from build123d import *

# Parameters (mm, degrees)
F0_R     = 1.5
F1_DEPTH = 2
F2_R     = 5


with BuildPart() as f1:
    # F0 (on Top) → F1 (new body)
    with BuildSketch(Plane.XY):
        with BuildLine():
            add(Edge.make_bspline(
                [(-13.142859, 26.857141), (-8.951076, 24.20284), (-4.564468, 21.895542), (0, 20)],
                knots=[66.18026, 66.18026, 66.18026, 66.18026, 80.865454, 80.865454, 80.865454, 80.865454], degree=3))
            Line((-13.142859, 26.857141), (-20, 20))
            Line((-20, 20), (-26.857141, 13.142859))
            add(Edge.make_bspline(
                [(-26.857141, 13.142859), (-24.20284, 8.951076), (-21.895542, 4.564468), (-20, 0)],
                knots=[66.18026, 66.18026, 66.18026, 66.18026, 80.865454, 80.865454, 80.865454, 80.865454], degree=3))
            Line((-20, 0), (-14.625, 0))
            Line((-14.625, 0), (-14.625, 6.5))
            Line((-14.625, 6.5), (-12.875, 6.5))
            Line((-12.875, 6.5), (-12.875, 0))
            Line((-12.875, 0), (0, 0))
            Line((0, 0), (0, 20))
        make_face()
        with Locations((-18, 6.25)):
            Circle(F0_R, mode=Mode.SUBTRACT)
        with Locations((-7.5, 7.5)):
            Circle(F0_R, mode=Mode.SUBTRACT)
        with Locations((-6.25, 18)):
            Circle(F0_R, mode=Mode.SUBTRACT)
        with BuildLine():
            Line((-14.625, 0), (-20, 0))
            add(Edge.make_bspline(
                [(-26.854903, -13.145097), (-24.198754, -8.951027), (-21.891877, -4.563394), (-20, 0)],
                knots=[66.166, 66.166, 66.166, 66.166, 80.865454, 80.865454, 80.865454, 80.865454], degree=3))
            Line((-26.854903, -13.145097), (-20, -20))
            Line((-20, -20), (-13.145097, -26.854903))
            add(Edge.make_bspline(
                [(0, -20), (-4.563394, -21.891877), (-8.951027, -24.198754), (-13.145097, -26.854903)],
                knots=[0, 0, 0, 0, 14.699453, 14.699453, 14.699453, 14.699453], degree=3))
            Line((0, -20), (0, 0))
            Line((0, 0), (-12.875, 0))
            Line((-12.875, 0), (-12.875, -6.5))
            Line((-12.875, -6.5), (-14.625, -6.5))
            Line((-14.625, -6.5), (-14.625, 0))
        make_face()
        with Locations((-6.25, -18)):
            Circle(F0_R, mode=Mode.SUBTRACT)
        with Locations((-18, -6.25)):
            Circle(F0_R, mode=Mode.SUBTRACT)
        with Locations((-7.5, -7.5)):
            Circle(F0_R, mode=Mode.SUBTRACT)
        with BuildLine():
            Line((-11.161165, 28.838835), (-13.142859, 26.857141))
            add(Edge.make_bspline(
                [(-13.142859, 26.857141), (-8.951076, 24.20284), (-4.564468, 21.895542), (0, 20)],
                knots=[66.18026, 66.18026, 66.18026, 66.18026, 80.865454, 80.865454, 80.865454, 80.865454], degree=3))
            add(Edge.make_bspline(
                [(13.145097, 26.854903), (8.951027, 24.198754), (4.563394, 21.891877), (0, 20)],
                knots=[66.166, 66.166, 66.166, 66.166, 80.865454, 80.865454, 80.865454, 80.865454], degree=3))
            Line((13.145097, 26.854903), (11.161165, 28.838835))
            add(Edge.make_bspline(
                [(-11.161165, 28.838835), (-7.440777, 25.169417), (0, 17.830583), (7.440777, 25.169417), (11.161165, 28.838835)],
                knots=[0, 0, 0, 0, 13.357773, 26.715546, 26.715546, 26.715546, 26.715546], degree=3))
        make_face()
        with BuildLine():
            add(Edge.make_bspline(
                [(-26.857141, 13.142859), (-24.20284, 8.951076), (-21.895542, 4.564468), (-20, 0)],
                knots=[66.18026, 66.18026, 66.18026, 66.18026, 80.865454, 80.865454, 80.865454, 80.865454], degree=3))
            Line((-26.857141, 13.142859), (-28.838835, 11.161165))
            add(Edge.make_bspline(
                [(-28.838835, -11.161165), (-25.169417, -7.440777), (-17.830583, 0), (-25.169417, 7.440777), (-28.838835, 11.161165)],
                knots=[0, 0, 0, 0, 13.357773, 26.715546, 26.715546, 26.715546, 26.715546], degree=3))
            Line((-28.838835, -11.161165), (-26.854903, -13.145097))
            add(Edge.make_bspline(
                [(-26.854903, -13.145097), (-24.198754, -8.951027), (-21.891877, -4.563394), (-20, 0)],
                knots=[66.166, 66.166, 66.166, 66.166, 80.865454, 80.865454, 80.865454, 80.865454], degree=3))
        make_face()
        with BuildLine():
            Line((28.838835, 11.161165), (26.854903, 13.145097))
            add(Edge.make_bspline(
                [(26.854903, 13.145097), (24.198754, 8.951027), (21.891877, 4.563394), (20, 0)],
                knots=[66.166, 66.166, 66.166, 66.166, 80.865454, 80.865454, 80.865454, 80.865454], degree=3))
            add(Edge.make_bspline(
                [(20, 0), (21.891877, -4.563394), (24.198754, -8.951027), (26.854903, -13.145097)],
                knots=[0, 0, 0, 0, 14.699454, 14.699454, 14.699454, 14.699454], degree=3))
            Line((26.854903, -13.145097), (28.838835, -11.161165))
            add(Edge.make_bspline(
                [(28.838835, 11.161165), (25.169417, 7.440777), (17.830583, 0), (25.169417, -7.440777), (28.838835, -11.161165)],
                knots=[0, 0, 0, 0, 13.357773, 26.715546, 26.715546, 26.715546, 26.715546], degree=3))
        make_face()
        with BuildLine():
            Line((12.875, 0), (0, 0))
            Line((0, 0), (0, -20))
            add(Edge.make_bspline(
                [(0, -20), (4.563394, -21.891877), (8.951027, -24.198754), (13.145097, -26.854903)],
                knots=[0, 0, 0, 0, 14.699453, 14.699453, 14.699453, 14.699453], degree=3))
            Line((13.145097, -26.854903), (20, -20))
            Line((20, -20), (26.854903, -13.145097))
            add(Edge.make_bspline(
                [(20, 0), (21.891877, -4.563394), (24.198754, -8.951027), (26.854903, -13.145097)],
                knots=[0, 0, 0, 0, 14.699454, 14.699454, 14.699454, 14.699454], degree=3))
            Line((20, 0), (14.625, 0))
            Line((14.625, 0), (14.625, -6.5))
            Line((14.625, -6.5), (12.875, -6.5))
            Line((12.875, -6.5), (12.875, 0))
        make_face()
        with Locations((6.25, -18)):
            Circle(F0_R, mode=Mode.SUBTRACT)
        with Locations((7.5, -7.5)):
            Circle(F0_R, mode=Mode.SUBTRACT)
        with Locations((18, -6.25)):
            Circle(F0_R, mode=Mode.SUBTRACT)
        with BuildLine():
            add(Edge.make_bspline(
                [(0, -20), (4.563394, -21.891877), (8.951027, -24.198754), (13.145097, -26.854903)],
                knots=[0, 0, 0, 0, 14.699453, 14.699453, 14.699453, 14.699453], degree=3))
            add(Edge.make_bspline(
                [(0, -20), (-4.563394, -21.891877), (-8.951027, -24.198754), (-13.145097, -26.854903)],
                knots=[0, 0, 0, 0, 14.699453, 14.699453, 14.699453, 14.699453], degree=3))
            Line((-13.145097, -26.854903), (-11.161165, -28.838835))
            add(Edge.make_bspline(
                [(11.161165, -28.838835), (7.440777, -25.169417), (0, -17.830583), (-7.440777, -25.169417), (-11.161165, -28.838835)],
                knots=[0, 0, 0, 0, 13.357773, 26.715546, 26.715546, 26.715546, 26.715546], degree=3))
            Line((11.161165, -28.838835), (13.145097, -26.854903))
        make_face()
        with BuildLine():
            add(Edge.make_bspline(
                [(13.145097, 26.854903), (8.951027, 24.198754), (4.563394, 21.891877), (0, 20)],
                knots=[66.166, 66.166, 66.166, 66.166, 80.865454, 80.865454, 80.865454, 80.865454], degree=3))
            Line((0, 20), (0, 0))
            Line((0, 0), (12.875, 0))
            Line((12.875, 0), (12.875, 6.5))
            Line((12.875, 6.5), (14.625, 6.5))
            Line((14.625, 6.5), (14.625, 0))
            Line((14.625, 0), (20, 0))
            add(Edge.make_bspline(
                [(26.854903, 13.145097), (24.198754, 8.951027), (21.891877, 4.563394), (20, 0)],
                knots=[66.166, 66.166, 66.166, 66.166, 80.865454, 80.865454, 80.865454, 80.865454], degree=3))
            Line((26.854903, 13.145097), (20, 20))
            Line((20, 20), (13.145097, 26.854903))
        make_face()
        with Locations((7.5, 7.5)):
            Circle(F0_R, mode=Mode.SUBTRACT)
        with Locations((18, 6.25)):
            Circle(F0_R, mode=Mode.SUBTRACT)
        with Locations((6.25, 18)):
            Circle(F0_R, mode=Mode.SUBTRACT)
    extrude(amount=F1_DEPTH)

    # F2
    f2_edges = [f1.edges().sort_by_distance(p)[0] for p in [
        (-11.161165, 28.838835, 1),
        (-28.838835, 11.161165, 1),
        (11.161165, 28.838835, 1),
        (28.838835, 11.161165, 1),
        (28.838835, -11.161165, 1),
        (11.161165, -28.838835, 1),
        (-11.161165, -28.838835, 1),
        (-28.838835, -11.161165, 1),
    ]]
    fillet(f2_edges, radius=F2_R)


solid = f1.part
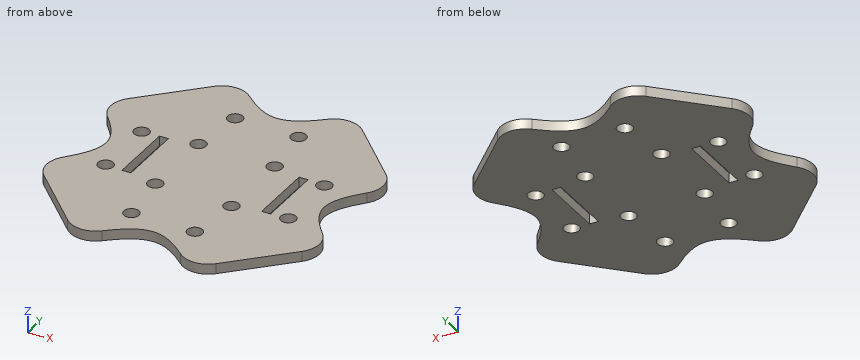
Geometry: final body of the model. Coordinates: model frame, mm. Coordinates: 2 decimals unless noted, no trailing zeros. Order: outer loops, then holes, each group sorted by start corner. A loop starts at its lowest first (then second) coordinate and runs counter-clockwise, first axis right, second up.
(1) Material intervals for probe 1 along X at (y, z) = (-1, 0.55) (3 decimals); probe 2 along X at (y, z) = (-7, 0.45); probe 3 along Y at (x, z) = (17.5, 1.05), sorted ascending.
(2) Section query C-C (z = 0.55). State how many separate pieces and enclosed holes the cut face has, plus the area to 3 significant figures.
(3) Section query A-A (x = -18). Return the cut outline in (y, z), plus the area to 3 significant figures.
(4) First-contact query: pin 1 (0.9 mm diameter, centred on x = 13.5, z = 1, fed in from +Y); pin 2 (0.9 mm diameter, centred on x = 14, z = 1, fed in from -Y). Flat tips, straight axial feed; report the tip coordinate or a pass-through.
Solution:
1. probe 1: x = -21.586 to -14.625, -12.875 to 12.875, 14.625 to 21.586
1. probe 2: x = -24.92 to -19.3, -16.7 to -8.91, -6.09 to 6.09, 8.91 to 16.7, 19.3 to 24.92
1. probe 3: y = -22.5 to -7.66, -4.84 to 4.84, 7.66 to 22.5
2. separate pieces: 1
2. enclosed holes: 14
2. area: 2,120 mm2
3. outline: (-22, 0) - (-7.75, 0) - (-7.75, 2) - (-22, 2) - close; (-4.75, 0) - (4.75, 0) - (4.75, 2) - (-4.75, 2) - close; (7.75, 0) - (22, 0) - (22, 2) - (7.75, 2) - close
3. area: 76.0 mm2
4. pin 1: stops at y = 26.44
4. pin 2: stops at y = -26.2
